```python
from build123d import *

# Parameters (mm, degrees)
SKETCH_1_R               = 16
EXTRUDE_1_DEPTH          = 54
FILLET_1_R               = 7
SHELL_1_T                = -2
CUT_EXTRUDE_1_DEPTH      = 59.549124673
CUT_EXTRUDE_1_DEPTH_BACK = 59.549124673
SKETCH_3_W               = 17.994708596
SKETCH_3_H               = 55.587571792
SKETCH_4_W               = 8
SKETCH_4_H               = 16.979772428
CUT_EXTRUDE_3_DEPTH      = 22
SKETCH_5_W               = 8
SKETCH_5_H               = 16.394935261
CUT_EXTRUDE_4_DEPTH      = 5
EXTRUDE_2_REACH          = 59.035
EXTRUDE_2_END_RADIUS     = 14
SKETCH_6_R               = 7
SKETCH_8_R               = 6.4
CUT_EXTRUDE_6_DEPTH      = 2
CUT_EXTRUDE_6_DRAFT      = -30
SKETCH_10_W              = 0.8
SKETCH_10_H              = 8
SKETCH_10_W_2            = 3.15
SKETCH_10_H_2            = 0.8
SKETCH_10_W_3            = 2.5
SKETCH_10_H_3            = 18
CUT_EXTRUDE_7_DEPTH      = 2
EXTRUDE_3_DEPTH          = 3.7
EXTRUDE_3_DEPTH_BACK     = 2
SKETCH_7_R               = 2.5
HOLE_WIZARD_M3_1_D       = 3.4
FILLET_3_R               = 2


with BuildPart() as part:
    # 스케치1 → 보스-돌출1 (new body)
    with BuildSketch(Plane(origin=(0, 0, 0), x_dir=(1, 0, 0), z_dir=(0, 1, 0))):
        with Locations(Location((0, 0, 0), (0, 0, 270))):
            Circle(SKETCH_1_R)
    extrude(amount=EXTRUDE_1_DEPTH)

    # 스케치2 → 컷-회전1 (revolve, cut)
    with BuildSketch(Plane.XY, mode=Mode.PRIVATE) as cut_revolve_1_sk:
        Polygon((19.244798042, 14.9), (13.5, 14.9), (13.5, 12), (8, 12), (8, 4.6), (10.65, 2.4), (10.65, 0), (19.244798042, 0), align=None)
    revolve(cut_revolve_1_sk.sketch.rotate(Axis((0, 0, 0), (0, 1, 0)), 90), axis=Axis((0, 0, 0), (0, 1, 0)), mode=Mode.SUBTRACT)

    # 필렛1
    fillet_1_edges = [part.edges().sort_by_distance(p)[0] for p in [
        (0, 54, -16),
    ]]
    fillet(fillet_1_edges, radius=FILLET_1_R)

    # 쉘1
    shell_1_openings = [part.faces().sort_by_distance(p)[0] for p in [
        (0, 0, 0),
    ]]
    offset(amount=SHELL_1_T, openings=shell_1_openings, kind=Kind.INTERSECTION)

    # 스케치3 → 컷-돌출1 (cut, two sides: drawn at the far end of the back side and taken through both)
    with BuildSketch(Plane.XY.offset(-CUT_EXTRUDE_1_DEPTH_BACK)):
        with Locations((8.997354298, 27.793785896)):
            Rectangle(SKETCH_3_W, SKETCH_3_H)
    extrude(amount=CUT_EXTRUDE_1_DEPTH + CUT_EXTRUDE_1_DEPTH_BACK, mode=Mode.SUBTRACT)

    # 스케치4 → 컷-돌출3 (cut)
    with BuildSketch(Plane(origin=(0, 54, 0), x_dir=(1, 0, 0), z_dir=(0, 1, 0))):
        with Locations((-4, -8.489886214)):
            Rectangle(SKETCH_4_W, SKETCH_4_H)
    extrude(amount=-CUT_EXTRUDE_3_DEPTH, mode=Mode.SUBTRACT)

    # 스케치5 → 컷-돌출4 (cut)
    with BuildSketch(Plane(origin=(0, 54, 0), x_dir=(1, 0, 0), z_dir=(0, 1, 0))):
        with Locations((-4, 8.197467631)):
            Rectangle(SKETCH_5_W, SKETCH_5_H)
    extrude(amount=-CUT_EXTRUDE_4_DEPTH, mode=Mode.SUBTRACT)

    # 보스-돌출2: up to this cylinder (the profile starts inside it)
    extrude_2_end = Plane(origin=(0, 45, 0), z_dir=(0, -1, 0)) * Cylinder(EXTRUDE_2_END_RADIUS, 147.07, mode=Mode.PRIVATE)
    # 스케치6 → 보스-돌출2 (add, up to the surface)
    with BuildSketch(Plane(origin=(-9, 0, 0), x_dir=(0, 0, -1), z_dir=(1, 0, 0)), mode=Mode.PRIVATE) as extrude_2_sk1:
        with Locations((0, 45)):
            Circle(SKETCH_6_R)
    extrude_2_tool1 = extrude(extrude_2_sk1.sketch, amount=-EXTRUDE_2_REACH, mode=Mode.PRIVATE) & extrude_2_end
    add(extrude_2_tool1.solids().sort_by_distance((-9, 45, 0))[0])


with BuildPart() as cut_extrude_6_tool:
    # 스케치8 → 컷-돌출6 (with draft: the straight prism first)
    with BuildSketch(Plane(origin=(-9, 0, 0), x_dir=(0, 0, -1), z_dir=(1, 0, 0))):
        with Locations((0, 45)):
            Circle(SKETCH_8_R)
    extrude(amount=-CUT_EXTRUDE_6_DEPTH)
    # 컷-돌출6: the draft: its side faces are tilted about the plane it starts from
    cut_extrude_6_sides = [cut_extrude_6_tool.faces().sort_by_distance(p)[0] for p in [
        (-10, 45, 6.4),
    ]]
    draft(cut_extrude_6_sides, Plane(origin=(-9, 0, 0), x_dir=(0, 0, -1), z_dir=(1, 0, 0)), CUT_EXTRUDE_6_DRAFT)


with BuildPart() as part_1:
    add(part.part)

    # 컷-돌출6: cut by cut_extrude_6_tool
    add(cut_extrude_6_tool.part, mode=Mode.SUBTRACT)

    # 스케치10 → 컷-돌출7 (cut)
    with BuildSketch(Plane(origin=(0, 0, 0), x_dir=(0, 0, -1), z_dir=(1, 0, 0))):
        with Locations((-14.25, 22.5)):
            Rectangle(SKETCH_10_W, SKETCH_10_H)
        with Locations((-13.075, 16.5)):
            Rectangle(SKETCH_10_W_2, SKETCH_10_H_2)
        with Locations((12.75, 16.5)):
            Rectangle(SKETCH_10_W_3, SKETCH_10_H_2)
        with Locations((14.25, 27.5)):
            Rectangle(SKETCH_10_W, SKETCH_10_H_3)
    extrude(amount=-CUT_EXTRUDE_7_DEPTH, mode=Mode.SUBTRACT)

    # 스케치7 → 보스-돌출3 (add, two sides: drawn at the far end of the back side and taken through both)
    with BuildSketch(Plane(origin=(-9, 0, 0), x_dir=(0, 0, -1), z_dir=(1, 0, 0)).offset(-EXTRUDE_3_DEPTH_BACK)):
        with Locations((0, 45)):
            Circle(SKETCH_7_R)
    extrude(amount=EXTRUDE_3_DEPTH + EXTRUDE_3_DEPTH_BACK)

    # M3 여유 구멍1 (through all)
    with Locations(Plane(origin=(-5.3, 45, 0), x_dir=(0, 0, 1), z_dir=(1, 0, 0))):
        with Locations((0, 0)):
            Hole(HOLE_WIZARD_M3_1_D / 2)

    # 필렛3
    fillet_3_edges = [part_1.edges().sort_by_distance(p)[0] for p in [
        (-11, 45, 2.5),
    ]]
    fillet(fillet_3_edges, radius=FILLET_3_R)


solid = part_1.part
```
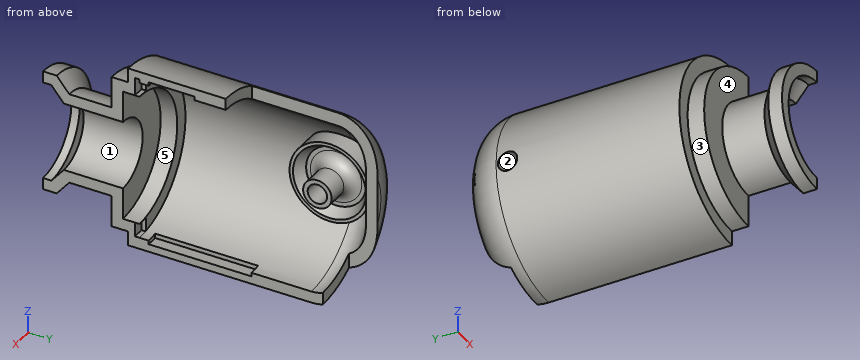
Input: part model. Units: mm. Frame: model coordinates. Face numbers are marked on the shaded views. A direction names the side the tool comes from. Round coordinates to 2 decimals unless told otherwise and drop trailing zeros. Loops run counter-clockwise (first coordinate to the right, second up) from the corner with the lowest first, then second, coordinate; pieces in that order, holes last. Notation, with made-up numbers: (9.5, 16.25) - (51.5, 16.25) arc R25 cw to (51.5, 46.25) - close; hole circle Ø3 at (74.5, 66.5). An arc over 180 degrees is marked (long way). One line per item, written item: value. Start each with the question number.
(1) Access query for the marked faces 3, 4 and 5. Directions: +Z, -Z, +X, -X, +Y, -Y. A direction counts if a zero-diameter tool reaches every point of the face in a straight line with its end or side. Return the directions, or none.
(2) Section A-A, the plane y = 34. Return loops of the section in (x, z).
(3) Section B-B, the plane y = 45. Return loops of the section in (x, z), plus the area to 3 significant figures.
(4) Draft query along Y for the marked faces 1 and 2. Return one class per face: +Y half, -Y half, draft (parallel to the pull), parting line (faces both ways), or undercut.
(5) Section C-C, the plane y = 28. Return loops of the section in (x, z).
(6) Ray query, line 1 (Y direction, x = -7.75, z = 0); line 2 (Y direction, x = -8.75, z = 0); line 3 (Z direction, x = -9.5, y = 45). Return the intervals inside material, ascending. Write a range as [from, to].
(7) Section D-D, the plane y = 22. Return loops of the section in (x, z), plus the area to 3 significant figures.
(8) Contact query for flat-ended pins moving along their axis: P1, Ø1.5, axis at x = -6, z = -8.5, coming from the -Y side; P2, Ø8, axis at x = -8.5, y = 21.5, coming from the +Z side; P3, Ø0.6, axis at x = -1, z = -14, coming from the -Y side; P4, Ø0.6, axis at x = -1, y = 16.5, coming from the +Z side. Output: stop coordinate, or through.
Results below:
1. face 3: -X, -Y
1. face 4: -X
1. face 5: +X
2. outline: (-8, 11.49) - (-8, 13.86) arc R16 ccw to (0, -16) - (0, -14.65) - (-2, -14.65) - (-2, -13.86) arc R14 cw to start
3. outline: (-15.91, -1.7) arc R16 ccw to (0, -16) - (0, -14) arc R14 cw to (-12.12, -7) - (-9, -7) - (-9, -6.4) - (-11, -5.25) - (-11, -4.5) arc R2 cw to (-9, -2.5) - (-5.3, -2.5) - (-5.3, -1.7) - close; (-15.91, 1.7) - (-5.3, 1.7) - (-5.3, 2.5) - (-9, 2.5) arc R2 cw to (-11, 4.5) - (-11, 5.25) - (-9, 6.4) - (-9, 7) - (-12.12, 7) arc R14 cw to (-8, 11.49) - (-8, 13.86) arc R16 ccw to start
3. area: 110 mm^2
4. face 1: draft
4. face 2: undercut
5. outline: (-2, -14.65) - (-2, -13.86) arc R14 cw to (0, 14) - (0, 16) arc R16 ccw to (0, -16) - (0, -14.65) - close
6. line 1: [2.21, 14], [42.5, 43.3], [46.7, 47.5]
6. line 2: [0, 3.98], [12, 14], [42.5, 43.3], [46.7, 47.5], [52, 54]
6. line 3: [-12.87, -10.28], [-7, -6.11], [-2.56, -1.7], [1.7, 2.56], [6.11, 7], [10.28, 12.87]
7. outline: (-2, -14.65) - (-2, -13.86) arc R14 cw to (-2, 13.86) - (-2, 14.65) - (0, 14.65) - (0, 16) arc R16 ccw to (0, -16) - (0, -14.65) - close
7. area: 91.5 mm^2
8. P1: y = 0
8. P2: z = 15.35
8. P3: y = 14.9
8. P4: z = 15.98
